The figure shows three views and two pictorial views of one solid part (mm, origin at its lowest corner). Answer the questions. A direction names the side the tool comes from. Round coordinates to 2 decimals unless told otherwise and drop trailing zeros. Order: outer loops, then holes, each group sorted by start corner. A loop starts at its lowest first (then second) coordinate and runs counter-clockwise, first axis right, second up. Notation, with made-up numbers: M -26.75,56 L 11.25,56 A14 ccw 11.25,70 Z; hole C 11,-7 d3. An arc over 180 degrees is marked long. Answer as CSV lines item,"result".
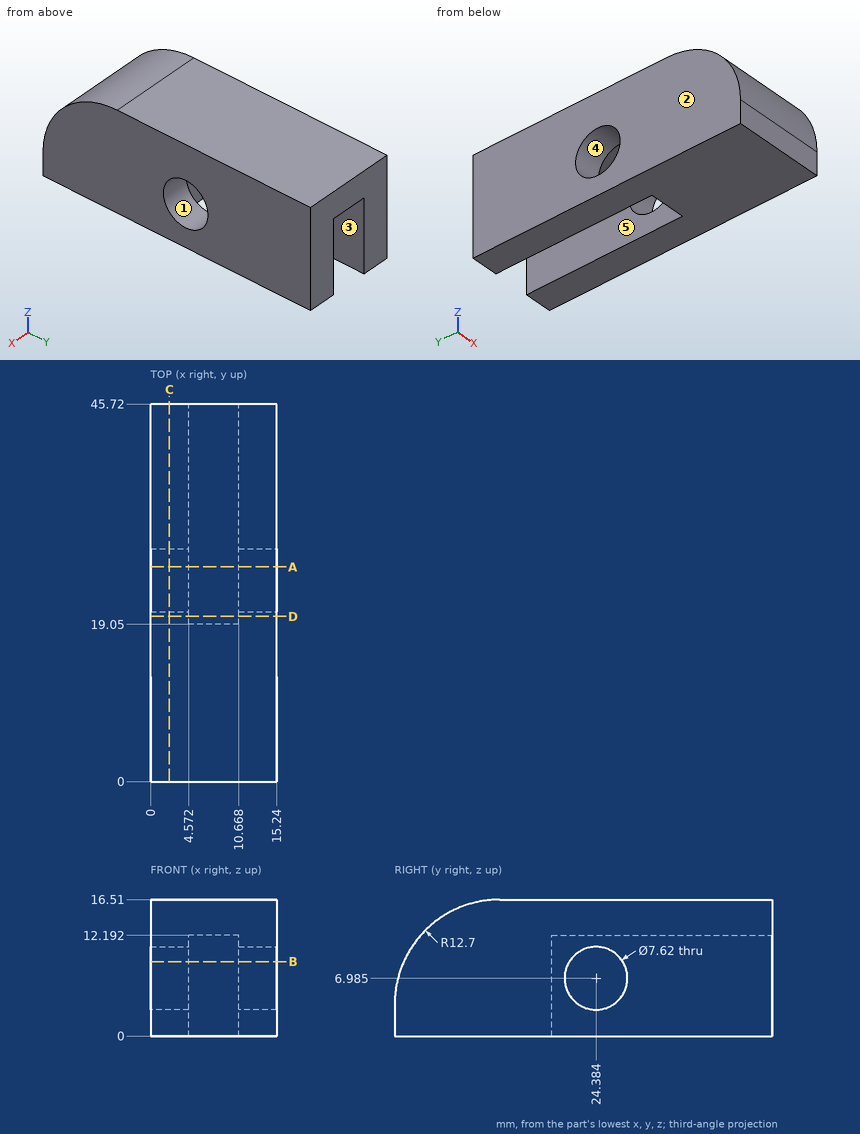
Item 1: Determine the mould class of the marked faces 1, 2 and 3 for opening direction X: +X half, -X half, draft (parallel to the pull), parting line (faces both ways), or undercut.
Ans:
face 1,"draft"
face 2,"-X half"
face 3,"undercut"
Item 2: A cutting plane is placed at C-C, the plane x = 2.25. Determine the outline of the cut face in (y, z) (3 decimals), and give its area (3 significant figures).
Ans:
outline,"M 0,0 L 45.72,0 L 45.72,16.51 L 12.7,16.51 A12.7 ccw 0,3.81 Z; hole C 24.384,6.985 d7.62"
area,"675 mm2"
Item 3: A cutting plane is placed at A-A, the plane y = 26. Determine the outline of the cut face in (x, z), and give its area (3 significant figures).
Ans:
outline,"M 0,0 L 4.57,0 L 4.57,3.53 L 0,3.53 Z; M 0,10.44 L 4.57,10.44 L 4.57,12.19 L 10.67,12.19 L 10.67,10.44 L 15.24,10.44 L 15.24,16.51 L 0,16.51 Z; M 10.67,0 L 15.24,0 L 15.24,3.53 L 10.67,3.53 Z"
area,"114 mm2"
Item 4: A cutting plane is placed at B-B, the plane z = 9. Determine the outline of the cut face in (x, y).
Ans:
outline,"M 0,1.11 L 15.24,1.11 L 15.24,21.15 L 10.67,21.15 L 10.67,19.05 L 4.57,19.05 L 4.57,21.15 L 0,21.15 Z; M 0,27.62 L 4.57,27.62 L 4.57,45.72 L 0,45.72 Z; M 10.67,27.62 L 15.24,27.62 L 15.24,45.72 L 10.67,45.72 Z"
Item 5: Flat-ended cylindrical pins translate along their axes: pin 1 (2 mm diameter, centred on x = 9.5, z = 11, fed in from -Y); pin 2 (3 mm diameter, centred on x = 9, y = 32, fed in from -Z); pin 3 (3 mm diameter, centred on x = 8.5, z = 4, fed in from +Y). Find the tip coordinate at first contact, or state that the pin passes through.
Ans:
pin 1,"y = 1.61"
pin 2,"z = 12.19"
pin 3,"y = 19.05"
Item 6: A tool of negligible diameter and unlimited length cuts with its end or side. For the marked faces 4 and 5, from which of +Z, -Z, +X, -X, +Y, -Y can it reach the whole face along a straight path? Write none if from no direction.
Ans:
face 4,"+X, -X"
face 5,"-Z, +Y"
Item 7: Find the intervals of material crossed by probe 1 along Z at (x, y) = (6, 43); probe 2 along X at (y, z) = (42.5, 9.5); probe 3 along Y at (x, z) = (8, 2), in increasing order. Write a range as [from, to].
Ans:
probe 1,"[12.19, 16.51]"
probe 2,"[0, 4.57], [10.67, 15.24]"
probe 3,"[0, 19.05]"
Item 8: A cutting plane is placed at D-D, the plane y = 20. Determine the outline of the cut face in (x, z).
Ans:
outline,"M 0,0 L 4.57,0 L 4.57,12.19 L 10.67,12.19 L 10.67,0 L 15.24,0 L 15.24,16.51 L 0,16.51 Z"
